from build123d import *

# Parameters (mm, degrees)
HIB_BASE_DEPTH        = 7.05
SKETCH1_3_R           = 3.5
LEG_JOINT_DEPTH       = 0.75
SKETCH2_R             = 1.2
LEG_PEG_DEPTH         = 2.4
LEG_PEG_INNER_DEPTH   = 1.2
LEG_LOCK_DEPTH        = 0.7
HIP_PEG_DEPTH         = 4.8
HIP_CAVITY_DEPTH      = 4.8
HIP_PEG_CHAMFER_DEPTH = 4.9


with BuildPart() as part:
    # Sketch1 → Hib Base (new body, symmetric)
    with BuildSketch(Plane(origin=(0, 0, 0), x_dir=(0, 0, -1), z_dir=(1, 0, 0))):
        with BuildLine():
            ThreePointArc((-2.343074903, -2.1), (0, -1.2), (2.343074903, -2.1))
            Line((2.343074903, -2.1), (3.9, -2.1))
            Line((3.9, -2.1), (3.9, 0))
            Line((3.9, 0), (-3.9, 0))
            Line((-3.9, 0), (-3.9, -2.1))
            Line((-3.9, -2.1), (-2.343074903, -2.1))
        make_face()
    extrude(amount=HIB_BASE_DEPTH, both=True)

    # Sketch1<3> → Leg Joint (add, symmetric)
    with BuildSketch(Plane(origin=(0, 0, 0), x_dir=(0, 0, -1), z_dir=(1, 0, 0))):
        with Locations((0, -4.7)):
            Circle(SKETCH1_3_R)
    extrude(amount=LEG_JOINT_DEPTH, both=True)

    # Sketch2 → Leg Peg (add)
    with BuildSketch(Plane(origin=(0.75, 0, 0), x_dir=(0, 0, -1), z_dir=(1, 0, 0))):
        with Locations((0, -4.7)):
            Circle(SKETCH2_R)
    leg_peg = extrude(amount=LEG_PEG_DEPTH)

    # Sketch3 → Leg Peg Inner (add)
    with BuildSketch(Plane(origin=(3.15, 0, 0), x_dir=(0, 0, -1), z_dir=(1, 0, 0))):
        with BuildLine():
            Line((-0.661437828, -3.95), (0.661437828, -3.95))
            ThreePointArc((0.661437828, -3.95), (0, -5.7), (-0.661437828, -3.95))
        make_face()
    leg_peg_inner = extrude(amount=LEG_PEG_INNER_DEPTH)

    # Sketch4 → Leg Lock (add)
    with BuildSketch(Plane(origin=(3.15, 0, 0), x_dir=(0, 0, -1), z_dir=(1, 0, 0))):
        with BuildLine():
            Line((-0.7, -5.8892855), (-0.7, -5.414142843))
            ThreePointArc((-0.7, -5.414142843), (0, -5.7), (0.7, -5.414142843))
            Line((0.7, -5.414142843), (0.7, -5.8892855))
            ThreePointArc((0.7, -5.8892855), (0, -6.08), (-0.7, -5.8892855))
        make_face()
    leg_lock = extrude(amount=LEG_LOCK_DEPTH)

    # Sketch5 → Hip Peg (add)
    with BuildSketch(Plane(origin=(0, 0, 0), x_dir=(1, 0, 0), z_dir=(0, 1, 0))):
        with BuildLine():
            ThreePointArc((1.55, -1), (2.539949494, -1.410050506), (2.95, -2.4))
            Line((2.95, -2.4), (4.95, -2.4))
            ThreePointArc((4.95, -2.4), (5.360050506, -1.410050506), (6.35, -1))
            Line((6.35, -1), (6.35, 1))
            ThreePointArc((6.35, 1), (5.360050506, 1.410050506), (4.95, 2.4))
            Line((4.95, 2.4), (2.95, 2.4))
            ThreePointArc((2.95, 2.4), (2.539949494, 1.410050506), (1.55, 1))
            Line((1.55, 1), (1.55, -1))
        make_face()
    hip_peg = extrude(amount=HIP_PEG_DEPTH)

    # Sketch6 → Hip Cavity (cut)
    with BuildSketch(Plane(origin=(0, 4.8, 0), x_dir=(1, 0, 0), z_dir=(0, 1, 0))):
        with BuildLine():
            Line((5.05, 0.866025404), (5.05, -0.866025404))
            ThreePointArc((5.05, -0.866025404), (2.55, 0), (5.05, 0.866025404))
        make_face()
    hip_cavity = extrude(amount=-HIP_CAVITY_DEPTH, mode=Mode.SUBTRACT)

    # Sketch7 → Hip Peg Chamfer (cut, symmetric)
    with BuildSketch(Plane.XY):
        Polygon((6.35, 4.8), (6.35, 1.8), (5.85, 4.8), align=None)
    hip_peg_chamfer = extrude(amount=HIP_PEG_CHAMFER_DEPTH, both=True, mode=Mode.SUBTRACT)

    # Mirror1: Leg Peg, Leg Peg Inner, Leg Lock, Hip Peg, Hip Cavity, Hip Peg Chamfer across plane
    add(leg_peg.mirror(Plane(origin=(0, 0, 0), x_dir=(0, 0, 1), z_dir=(1, 0, 0))))
    add(leg_peg_inner.mirror(Plane(origin=(0, 0, 0), x_dir=(0, 0, 1), z_dir=(1, 0, 0))))
    add(leg_lock.mirror(Plane(origin=(0, 0, 0), x_dir=(0, 0, 1), z_dir=(1, 0, 0))))
    add(hip_peg.mirror(Plane(origin=(0, 0, 0), x_dir=(0, 0, 1), z_dir=(1, 0, 0))))
    add(hip_cavity.mirror(Plane(origin=(0, 0, 0), x_dir=(0, 0, 1), z_dir=(1, 0, 0))), mode=Mode.SUBTRACT)
    add(hip_peg_chamfer.mirror(Plane(origin=(0, 0, 0), x_dir=(0, 0, 1), z_dir=(1, 0, 0))), mode=Mode.SUBTRACT)


solid = part.part
The listing builds one solid part. Answer for the finished solid, in the listing's coordinates (mm). A direction names the side the tool comes from. Round coordinates to 2 decimals unless told otherwise and drop trailing zeros. Write each loop counter-clockwise with the first axis right and the second up, starting at its lowest first coordinate (ties: lowest second). Pieces come first, ordered by that corner, then holes. Notation, with made-up numbers: (47.25, 75) - (88.25, 75) arc R13 ccw to (88.25, 85) - close; hole circle Ø11 at (35, 3). An arc over 180 degrees is marked (long way). Use one line per item in the form item = value. Start each with the question number.
Item 1: A cutting plane is placed at C-C (y = -4.7). Write down the section's boundary in (x, z), plus the area to 3 significant figures.
Item 2: A tool of negligible diameter and unlimited length cuts with its end or side. For faces 4 (the flat face through (4, 2, -2.4)), 5 (the flat face through (-1.55, 2, 0)), 6 (the cylindrical face through (2.55, 2.43, 0.05)), 7 (the cylindrical face through (-1.93, -5.87, 0.26)), 8 (the cylindrical face through (2.53, 2.37, 1.4)), from which of +Z, -Z, +X, -X, +Y, -Y can it reach the whole face along a straight path? Write none if from no direction.
Item 3: A cutting plane is placed at A-A (y = 1.5). Write down the section's boundary in (x, z), plus the area to 3 significant figures.
Item 4: Determine the mould class of faces 1 (the flat face through (-4, 2, 2.4)), 2 (the cylindrical face through (-2.55, 2.37, -1.42)), 3 (the cylindrical face through (5.35, 2.37, 1.42)) for opening direction X: +X half, -X half, draft (parallel to the pull), parting line (faces both ways), or undercut.
Item 5: A cutting plane is placed at B-B (z = -3). Write down the section's boundary in (x, y).
Item 6: Find the intervals of material crossed by line 1 (X direction, y = 1.4, z = 0); line 2 (Z direction, x = -3.95, y = 1.7); line 3 (Y direction, x = 4.5, z = 2.5), in increasing order. Write a range as [from, to].
Item 7: Flat-ended cylindrical pins translate along their axes: pin 1 Ø0.5 at (y, z) = (-5.5, 0) entering from +X; pin 2 Ø3 at (x, z) = (-3.5, -1) entering from -Y; pin 3 Ø0.5 at (y, z) = (1.5, 0) entering from -X. Find the tip coordinate at first contact, or state that the pin passes through.
Item 8: A cutting plane is placed at D-D (x = 0). Write down the section's boundary in (y, z).
The answers:
q1.outline = (-4.35, -1) - (-3.15, -1) - (-3.15, -1.2) - (-0.75, -1.2) - (-0.75, -3.5) - (0.75, -3.5) - (0.75, -1.2) - (3.15, -1.2) - (3.15, -1) - (4.35, -1) - (4.35, 1) - (3.15, 1) - (3.15, 1.2) - (0.75, 1.2) - (0.75, 3.5) - (-0.75, 3.5) - (-0.75, 1.2) - (-3.15, 1.2) - (-3.15, 1) - (-4.35, 1) - close
q1.area = 26.8 mm^2
q2.face_4 = -Z, +X, -X, +Y
q2.face_5 = +Z, -Z, +Y
q2.face_6 = +Y
q2.face_7 = none
q2.face_8 = +Z, +Y
q3.outline = (-6.35, -1) arc R1.4 cw to (-4.95, -2.4) - (-2.95, -2.4) arc R1.4 cw to (-1.55, -1) - (-1.55, 1) arc R1.4 cw to (-2.95, 2.4) - (-4.95, 2.4) arc R1.4 cw to (-6.35, 1) - close; (1.55, -1) arc R1.4 cw to (2.95, -2.4) - (4.95, -2.4) arc R1.4 cw to (6.35, -1) - (6.35, 1) arc R1.4 cw to (4.95, 2.4) - (2.95, 2.4) arc R1.4 cw to (1.55, 1) - close; hole (-5.05, -0.87) arc R1.4 ccw (long way) to (-5.05, 0.87) - close; hole (5.05, -0.87) - (5.05, 0.87) arc R1.4 ccw (long way) to start
q3.area = 22.2 mm^2
q4.face_1 = draft
q4.face_2 = undercut
q4.face_3 = +X half
q5.outline = (-7.05, -2.1) - (7.05, -2.1) - (7.05, 0) - (-7.05, 0) - close; (-0.75, -6.5) - (0.75, -6.5) - (0.75, -2.9) - (-0.75, -2.9) - close
q6.line_1 = [-6.35, -5.05], [-2.55, -1.55], [1.55, 2.55], [5.05, 6.35]
q6.line_2 = [-2.4, -1.4], [1.4, 2.4]
q6.line_3 = [-2.1, 0]
q7.pin_1 = 4.35
q7.pin_2 = -6.08
q7.pin_3 = -6.35
q8.outline = (-2.1, -3.9) - (0, -3.9) - (0, 3.9) - (-2.1, 3.9) - (-2.1, 2.34) arc R3.5 ccw (long way) to (-2.1, -2.34) - close
